```python
from build123d import *

# Parameters (mm, degrees)
BOSS_EXTRUDE1_DEPTH = 26
CUT_EXTRUDE8_DEPTH  = 53
FILLET1_R           = 6
SKETCH2_R           = 2.9
SKETCH2_R_2         = 3.05
CUT_EXTRUDE1_DEPTH  = 29
SKETCH3_R           = 5.5
CUT_EXTRUDE2_DEPTH  = 7
CHAMFER2_SIZE       = 5
CUT_EXTRUDE9_DEPTH  = 53
CUT_EXTRUDE10_START = -5
CUT_EXTRUDE10_DEPTH = 4
FILLET2_R           = 5
SKETCH12_R          = 3.05
CUT_EXTRUDE11_DEPTH = 4
FILLET3_R           = 2


with BuildPart() as part:
    # Sketch1 → Boss-Extrude1 (new body, symmetric)
    with BuildSketch(Plane.XY):
        Polygon((35.4, 6), (-35.4, 6), (-35.4, -49.8), (-25.65, -49.8), (-25.65, -24.4), (25.65, -24.4), (25.65, -49.8), (35.4, -49.8), align=None)
    extrude(amount=BOSS_EXTRUDE1_DEPTH, both=True)

    # Sketch9 → Cut-Extrude8 (cut, through all)
    with BuildSketch(Plane.XY.offset(26)):
        Polygon((-30, 6), (-35.4, -14.65), (-35.4, 6), align=None)
        Polygon((35.4, 6), (30, 6), (35.4, -14.65), align=None)
    extrude(amount=-CUT_EXTRUDE8_DEPTH, mode=Mode.SUBTRACT)

    # Fillet1
    fillet1_edges = [part.edges().sort_by_distance(p)[0] for p in [
        (25.65, -24.4, 0),
        (-25.65, -24.4, 0),
    ]]
    fillet(fillet1_edges, radius=FILLET1_R)

    # Sketch2 → Cut-Extrude1 (cut)
    with BuildSketch(Plane(origin=(0, 6, 0), x_dir=(1, 0, 0), z_dir=(0, 1, 0))):
        with Locations((-23, 6.5)):
            Circle(SKETCH2_R)
        with Locations((-23, -6.5)):
            Circle(SKETCH2_R)
        with Locations((-15, 18.5)):
            Circle(SKETCH2_R_2)
        with Locations((23, -6.5)):
            Circle(SKETCH2_R)
        with Locations((23, 6.5)):
            Circle(SKETCH2_R)
        with Locations((15, 18.5)):
            Circle(SKETCH2_R_2)
        with Locations((15, -18.5)):
            Circle(SKETCH2_R_2)
        with Locations((-15, -18.5)):
            Circle(SKETCH2_R_2)
    extrude(amount=-CUT_EXTRUDE1_DEPTH, mode=Mode.SUBTRACT)

    # Sketch3 → Cut-Extrude2 (cut)
    with BuildSketch(Plane(origin=(0, 6, 0), x_dir=(1, 0, 0), z_dir=(0, 1, 0))):
        with Locations((-15, 18.5)):
            Circle(SKETCH3_R)
        with Locations((15, 18.5)):
            Circle(SKETCH3_R)
        with Locations((-15, -18.5)):
            Circle(SKETCH3_R)
        with Locations((15, -18.5)):
            Circle(SKETCH3_R)
    extrude(amount=-CUT_EXTRUDE2_DEPTH, mode=Mode.SUBTRACT)

    # Chamfer2
    chamfer2_edges = [part.edges().sort_by_distance(p)[0] for p in [
        (35.4, -49.8, 0),
        (-35.4, -49.8, 0),
    ]]
    chamfer(chamfer2_edges, length=CHAMFER2_SIZE)

    # Sketch10 → Cut-Extrude9 (cut, through all)
    with BuildSketch(Plane(origin=(0, 0, -26), x_dir=(-1, 0, 0), z_dir=(0, 0, -1))):
        with BuildLine():
            Line((-4.25, 0), (-4.25, 11.491510708))
            Line((-4.25, 11.491510708), (4.25, 11.491510708))
            Line((4.25, 11.491510708), (4.25, 0))
            ThreePointArc((4.25, 0), (0, -4.25), (-4.25, 0))
        make_face()
    extrude(amount=-CUT_EXTRUDE9_DEPTH, mode=Mode.SUBTRACT)

    # Sketch11 → Cut-Extrude10 (cut)
    with BuildSketch(Plane(origin=(0, 0, -26), x_dir=(-1, 0, 0), z_dir=(0, 0, -1)).offset(CUT_EXTRUDE10_START)):
        Polygon((-6.15, 3.550704156), (-6.15, 9.910448096), (6.15, 9.910448096), (6.15, 3.550704156), (6.15, -3.550704156), (0, -7.101408311), (-6.15, -3.550704156), align=None)
    extrude(amount=-CUT_EXTRUDE10_DEPTH, mode=Mode.SUBTRACT)

    # Fillet2
    fillet2_edges = [part.edges().sort_by_distance(p)[0] for p in [
        (4.25, 3, 26),
        (-4.25, 3, 26),
        (0, -4.25, 26),
    ]]
    fillet(fillet2_edges, radius=FILLET2_R)

    # Sketch12 → Cut-Extrude11 (cut)
    with BuildSketch(Plane(origin=(0, -23, 0), x_dir=(1, 0, 0), z_dir=(0, 1, 0))):
        with Locations((-15, 18.5)):
            Circle(SKETCH12_R)
        with Locations((15, 18.5)):
            Circle(SKETCH12_R)
        with Locations((15, -18.5)):
            Circle(SKETCH12_R)
        with Locations((-15, -18.5)):
            Circle(SKETCH12_R)
    extrude(amount=-CUT_EXTRUDE11_DEPTH, mode=Mode.SUBTRACT)

    # Fillet3
    fillet3_edges = [part.edges().sort_by_distance(p)[0] for p in [
        (-25.9, -23, -6.5),
        (20.1, -23, -6.5),
        (20.1, -23, 6.5),
        (-25.9, -23, 6.5),
    ]]
    fillet(fillet3_edges, radius=FILLET3_R)


solid = part.part
```
Source: CAD feature listing. Evaluate the final solid. Frame: model axes, mm. A direction names the side the tool comes from. Give positions to 0.01 mm unless a question says otherwise; leave off trailing zeros. Write each loop counter-clockwise with the first axis right and the second up, starting at its lowest first coordinate (ties: lowest second). Pieces come first, ordered by that corner, then holes. Notation, with made-up numbers: (-36.75, 55.5) - (-10.75, 55.5) arc R6 ccw to (-10.75, 59.5) - close; hole circle Ø4 at (31, 47.5). An arc over 180 degrees is marked (long way). One line per item, written item: value. Start each with the question number.
Q1. Section query D-D, the plane x = 15. Return the cut outline in (y, z).
Q2. Set-up query: faces 1 (the face through (-5.75, 3.04, 24.57)), 2 (the face through (16.64, -12.54, 15.93)), 3 (the face through (20.08, 2.55, 20.61)), 4 (the face through (25.65, -40, 0)), 5 (the face through (-0.09, -4.25, -23.54)). Return all of +Z, -Z, +X, -X, +Y, -Y with unobstructed straight access to the full face (end or side cutting, diameter ignored); none if empty.
Q3. Section query C-C, the plane z = -10.5. Return the cut outline in (x, y), then the cut area to 3 significant figures.
Q4. Section query B-B, the plane x = -17. Return the cut outline in (y, z).
Q5. First-contact query: pin 1 Ø12 at (x, z) = (-7.5, -1.5) entering from -Y; pin 2 Ø6.5 at (y, z) = (4, -3) entering from -X; pin 3 Ø0.9 at (x, z) = (-22.5, 6) entering from +Y. Flat tips, straight axial feed; report the tip coordinate or a pass-through.
Q6. Section query A-A, the plane y = -19.5. Count the separate pieces of the cut face and the enclosed holes in it, then the cut area to 3 significant figures.
Q7. Material intervals for probe 1 along Z at (x, y) = (-23, -11.5); probe 2 along X at (y, z) = (-7.5, -6.5); probe 3 along X at (y, z) = (-44.5, 14), sorted ascending. Write a range as from..to.
Q8. Draft query along X for faces 6 (the face through (17, -1, -16)), 7 (the face through (-28, -49.8, 0)). Return one class per face: +X half, -X half, draft (parallel to the pull), parting line (faces both ways), or undercut.
Answer:
1. outline: (-24.4, -26) - (6, -26) - (6, -24) - (-1, -24) - (-1, -21.55) - (-24.4, -21.55) - close; (-24.4, -15.45) - (-1, -15.45) - (-1, -13) - (6, -13) - (6, 13) - (-1, 13) - (-1, 15.45) - (-24.4, 15.45) - close; (-24.4, 21.55) - (-1, 21.55) - (-1, 24) - (6, 24) - (6, 26) - (-24.4, 26) - close
2. face 1: +Z, +Y
2. face 2: +Y, -Y
2. face 3: +Y
2. face 4: +Z, -Z, -Y
2. face 5: +Z, -Z, +Y
3. outline: (-35.4, -44.8) - (-30.4, -49.8) - (-25.65, -49.8) - (-25.65, -30.4) arc R6 cw to (-19.65, -24.4) - (19.65, -24.4) arc R6 cw to (25.65, -30.4) - (25.65, -49.8) - (30.4, -49.8) - (35.4, -44.8) - (35.4, -14.65) - (30, 6) - (4.25, 6) - (4.25, 0) arc R4.25 cw to (-4.25, 0) - (-4.25, 6) - (-30, 6) - (-35.4, -14.65) - close
3. area: 2,450 mm2
4. outline: (-24.4, -26) - (6, -26) - (6, -23.62) - (-1, -23.62) - (-1, -20.8) - (-24.4, -20.8) - close; (-24.4, -16.2) - (-1, -16.2) - (-1, -13.38) - (6, -13.38) - (6, 13.38) - (-1, 13.38) - (-1, 16.2) - (-24.4, 16.2) - close; (-24.4, 20.8) - (-1, 20.8) - (-1, 23.62) - (6, 23.62) - (6, 26) - (-24.4, 26) - close
5. pin 1: stops at y = -24.4
5. pin 2: stops at x = -31.37
5. pin 3: stops at y = -22.98
6. separate pieces: 1
6. enclosed holes: 8
6. area: 3,460 mm2
7. probe 1: z = -26..-9.4, -3.6..3.6, 9.4..26
7. probe 2: x = -33.53..-25.9, -20.1..20.1, 25.9..33.53
7. probe 3: x = -35.4..-25.65, 25.65..35.4
8. face 6: undercut
8. face 7: draft
